Can you work these out from the drawing? Everything is in mm from the part's minimum corner. A direction names the side the tool comes from. Coordinates: 2 decimals unless noted, no trailing zeros. Loops run counter-clockwise (first coordinate to the right, second up) from the corner with the lowest first, then second, coordinate; pieces in that order, holes last.
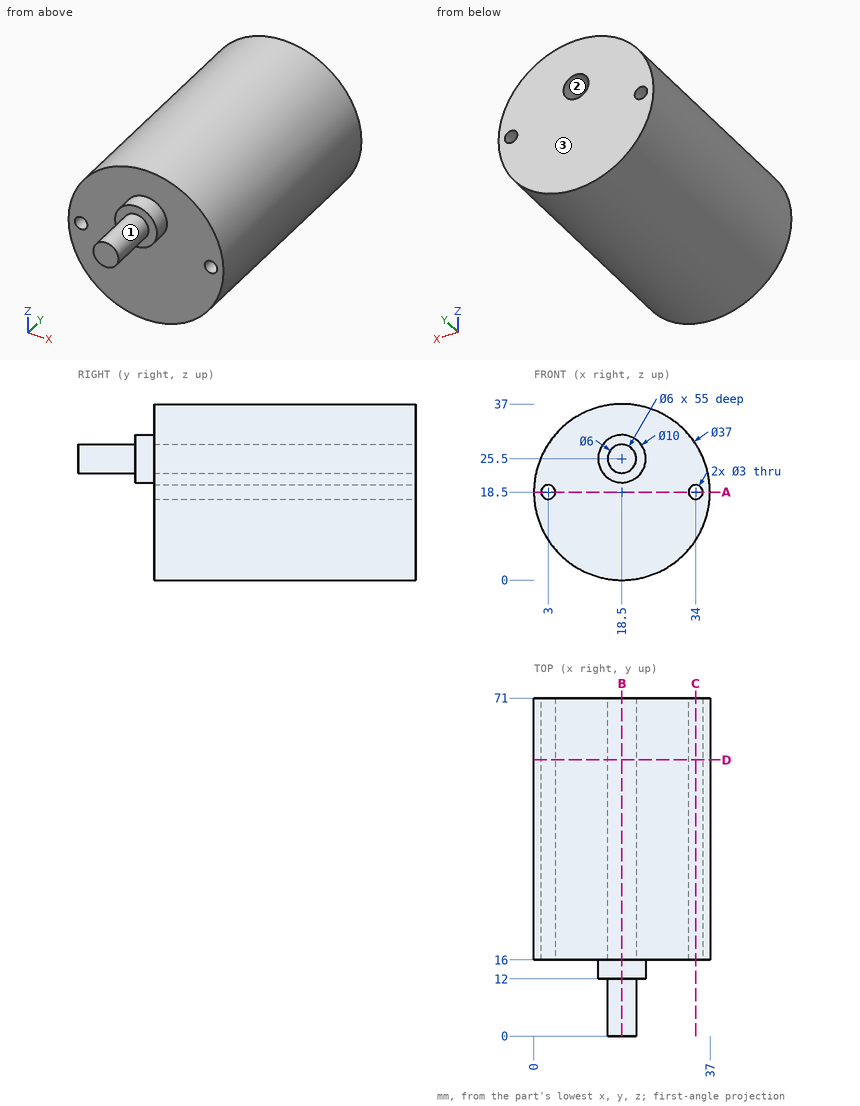
Item 1: I'm going to push flat-ended pins straight in: P1, Ø1.8, axis at x = 3, z = 18.5, coming from the +Y side; P2, Ø1.5, axis at x = 12, z = 15.5, coming from the -Y side; P3, Ø1, axis at x = 8.5, y = 60, coming from the -Z side; P4, Ø3, axis at x = 14, y = 25.5, coming from the +Z side. Where does each tip first touch, or does it pass through?
Results are:
P1: passes through
P2: stops at y = 16
P3: stops at z = 2.63
P4: stops at z = 36.76
Item 2: I need wall thicknesses on line 1 along X through (y, z) = (47, 18); line 2 along Y through (x, z) = (6.5, 23.5); line 3 along Z through (x, y) = (18.5, 59). Which ranges of each line are inside material? Lowest first, please.
Results are:
line 1: x = 0.01 to 1.59, 4.41 to 32.59, 35.41 to 36.99
line 2: y = 16 to 71
line 3: z = 0 to 22.5, 28.5 to 37
Item 3: Suppose I cut it at B-B, the plane x = 18.5. Please give me the cut outline in (y, z), plus the area to 3 significant figures.
Results are:
outline: (0, 22.5) - (12, 22.5) - (12, 20.5) - (16, 20.5) - (16, 0) - (71, 0) - (71, 22.5) - (16, 22.5) - (16, 28.5) - (71, 28.5) - (71, 37) - (16, 37) - (16, 30.5) - (12, 30.5) - (12, 28.5) - (0, 28.5) - close
area: 1,820 mm2
Item 4: On a 3-axis mill with a long thin cutter (end or side, diameter ignored), from which of +Z, -Z, +X, -X, +Y, -Y can I reach the whole of each face in a straight line? I mean the marked faces 1, 2 and 3. Say none if no direction works.
Results are:
face 1: -Y
face 2: +Y
face 3: +Z, -Z, +X, -X, +Y
Item 5: Suppose I cut it at D-D, the plane y = 58. Please give me the cut outline in (x, z), plus the area to 3 significant figures.
Results are:
outline: circle Ø37 at (18.5, 18.5); hole circle Ø3 at (3, 18.5); hole circle Ø6 at (18.5, 25.5); hole circle Ø3 at (34, 18.5)
area: 1,030 mm2
Item 6: Suppose I cut it at A-A, the plane z = 18.5. Please give me the cut outline in (x, y), plus the area to 4 significant figures.
Results are:
outline: (0, 16) - (1.5, 16) - (1.5, 71) - (0, 71) - close; (4.5, 16) - (32.5, 16) - (32.5, 71) - (4.5, 71) - close; (35.5, 16) - (37, 16) - (37, 71) - (35.5, 71) - close
area: 1,705 mm2
Item 7: Suppose I cut it at C-C, the plane x = 34. Please give me the cut outline in (y, z).
Results are:
outline: (16, 8.4) - (71, 8.4) - (71, 17) - (16, 17) - close; (16, 20) - (71, 20) - (71, 28.6) - (16, 28.6) - close
